The figure shows three views and two pictorial views of one solid part (mm, origin at its lowest corner). Answer the questions. Give positions to 0.01 mm unless a question says otherwise; leave off trailing zeros. Order: outer loops, then holes, each group sorted by start corner. A loop starts at its lowest first (then second) coordinate and runs counter-clockwise, first axis right, second up. Notation, with made-up numbers: (0, 30.25) -> (54, 30.25) arc R17 ccw to (54, 50.25) -> close; hole circle Ø11 at (-37.75, 20.25). An arc over 180 degrees is marked (long way). Use one line per item in the form item = value.
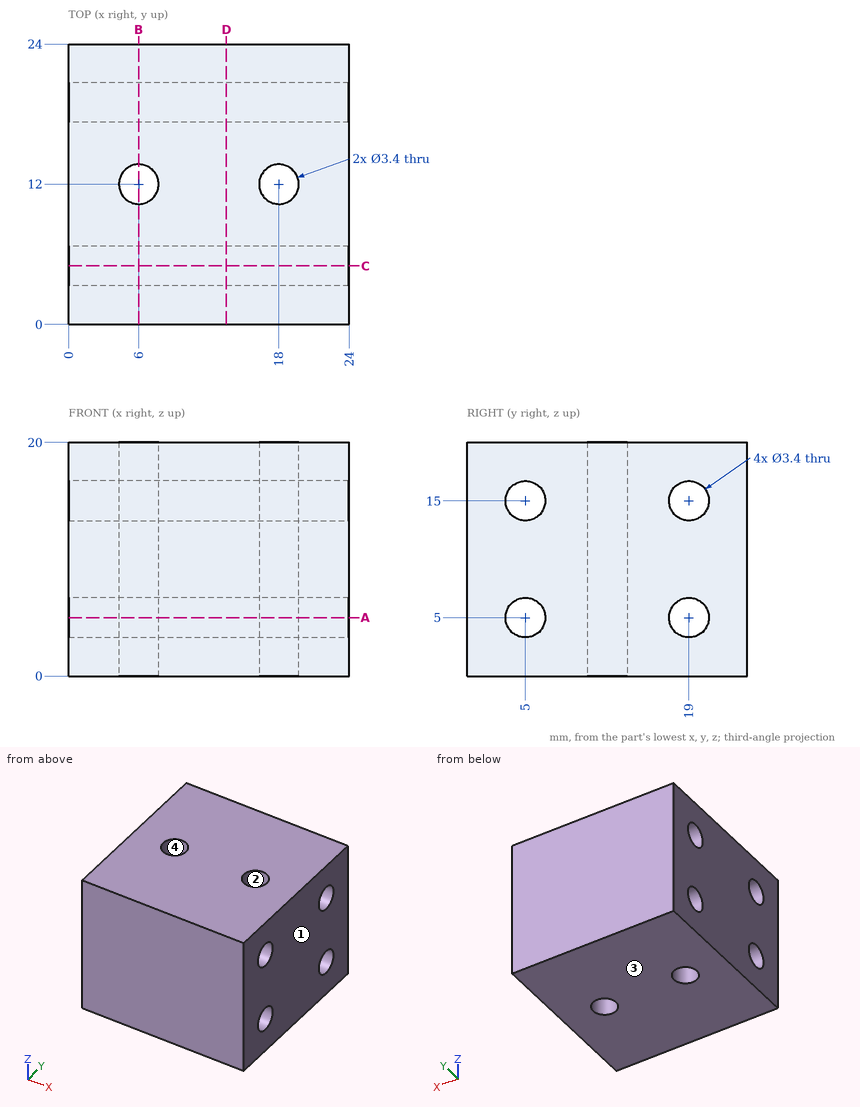
Item 1: The part is cut by section D-D on x = 13.5. Give the vertices of the cut face in (y, z).
Checks:
outline = (0, 0) -> (24, 0) -> (24, 20) -> (0, 20) -> close; hole circle Ø3.4 at (5, 5); hole circle Ø3.4 at (5, 15); hole circle Ø3.4 at (19, 5); hole circle Ø3.4 at (19, 15)
Item 2: Given pin 1 Ø3 at (y, z) = (19, 5) entering from +X; pin 2 Ø1.5 at (y, z) = (16, 8) entering from -X, each flat-ended and moving along its own axis, determine where each tip first touches the part or whether it passes through.
Checks:
pin_1 = through
pin_2 = 0
Item 3: The part is cut by section C-C on y = 5. Give the vertices of the cut face in (x, z), and give its area (3 significant figures).
Checks:
outline = (0, 0) -> (24, 0) -> (24, 3.3) -> (0, 3.3) -> close; (0, 6.7) -> (24, 6.7) -> (24, 13.3) -> (0, 13.3) -> close; (0, 16.7) -> (24, 16.7) -> (24, 20) -> (0, 20) -> close
area = 317 mm²
Item 4: The part is cut by section B-B on x = 6. Give the vertices of the cut face in (y, z).
Checks:
outline = (0, 0) -> (10.3, 0) -> (10.3, 20) -> (0, 20) -> close; (13.7, 0) -> (24, 0) -> (24, 20) -> (13.7, 20) -> close; hole circle Ø3.4 at (5, 5); hole circle Ø3.4 at (5, 15); hole circle Ø3.4 at (19, 5); hole circle Ø3.4 at (19, 15)
Item 5: The part is cut by section A-A on z = 5. Give the vertices of the cut face in (x, y), and give its area (3 significant figures).
Checks:
outline = (0, 0) -> (24, 0) -> (24, 3.3) -> (0, 3.3) -> close; (0, 6.7) -> (24, 6.7) -> (24, 17.3) -> (0, 17.3) -> close; (0, 20.7) -> (24, 20.7) -> (24, 24) -> (0, 24) -> close; hole circle Ø3.4 at (6, 12); hole circle Ø3.4 at (18, 12)
area = 395 mm²
Item 6: Straight lines are drawn through the part: L1, parallel to Y at x = 14.5, z = 5; L2, parallel to Z at x = 7.75, y = 5; L3, parallel to Z at x = 7.75, y = 18.5. For each, find the intervals that lie inside material, in ascending order. Write a range as from..to.
Checks:
L1 = 0..3.3, 6.7..17.3, 20.7..24
L2 = 0..3.3, 6.7..13.3, 16.7..20
L3 = 0..3.38, 6.62..13.38, 16.62..20
Item 7: Determine the mould class of the marked faces 1, 2, 3 and 4 for opening direction X: +X half, -X half, draft (parallel to the pull), parting line (faces both ways), or undercut.
Checks:
face_1 = +X half
face_2 = undercut
face_3 = draft
face_4 = undercut
